Build history of the part. All positions in model axes, mm. A direction names the side the tool comes from. Coordinates: 2 decimals unless noted, no trailing zeros. Order: outer loops, then holes, each group sorted by start corner. A loop starts at its lowest first (then second) coordinate and runs counter-clockwise, first axis right, second up. Notation, with made-up numbers: (22, -4) - (63, -4) arc R23 cw to (63, 24) - close; hole circle Ø11 at (28.5, 77). An arc over 180 degrees is marked (long way). One line per item, written item: value.
from build123d import *

# Parameters (mm, degrees)
F0_R     = 5
F0_W     = 15
F0_H     = 22
F1_DEPTH = 2.5


with BuildPart() as f1:
    # F0 (on Top) → F1 (new body)
    with BuildSketch(Plane.XY):
        with BuildLine():
            Line((30, 57), (-30, 57))
            ThreePointArc((-30, 57), (-33.535534, 55.535534), (-35, 52))
            Line((-35, 52), (-35, -52))
            ThreePointArc((-35, -52), (-33.535534, -55.535534), (-30, -57))
            Line((-30, -57), (30, -57))
            ThreePointArc((30, -57), (33.535534, -55.535534), (35, -52))
            Line((35, -52), (35, 52))
            ThreePointArc((35, 52), (33.535534, 55.535534), (30, 57))
        make_face()
        with Locations((0, -50.2)):
            Circle(F0_R, mode=Mode.SUBTRACT)
        Rectangle(F0_W, F0_H, mode=Mode.SUBTRACT)
        with Locations((0, 50.2)):
            Circle(F0_R, mode=Mode.SUBTRACT)
    extrude(amount=F1_DEPTH)


solid = f1.part
1. Band-saw the part on A-A, the plane y = 50.2. Give the cut face in (x, z), and give its area (3 significant figures).
Values found:
outline: (-35, 0) - (-5, 0) - (-5, 2.5) - (-35, 2.5) - close; (5, 0) - (35, 0) - (35, 2.5) - (5, 2.5) - close
area: 150 mm2
2. Band-saw the part on B-B, the plane x = -3. Give the cut face in (y, z), and give its area (3 significant figures).
Values found:
outline: (-57, 0) - (-54.2, 0) - (-54.2, 2.5) - (-57, 2.5) - close; (-46.2, 0) - (-11, 0) - (-11, 2.5) - (-46.2, 2.5) - close; (11, 0) - (46.2, 0) - (46.2, 2.5) - (11, 2.5) - close; (54.2, 0) - (57, 0) - (57, 2.5) - (54.2, 2.5) - close
area: 190 mm2
3. 3-axis set-ups, long thin cutter, end or side, ignore diameter. For faces 4 (the face through (34, 55, 1)), 5 (the face through (0, 11, 1)): which of +Z, -Z, +X, -X, +Y, -Y reach the whole face in a straight line?
Values found:
face 4: +Z, -Z, +X, +Y
face 5: +Z, -Z
4. Band-saw the part on D-D, the plane y = -8.5. Give the cut face in (x, z).
Values found:
outline: (-35, 0) - (-7.5, 0) - (-7.5, 2.5) - (-35, 2.5) - close; (7.5, 0) - (35, 0) - (35, 2.5) - (7.5, 2.5) - close
5. Band-saw the part on C-C, the plane z = 1.1. Give the cut face in (x, y), and give its area (3 significant figures).
Values found:
outline: (-35, -52) arc R5 ccw to (-30, -57) - (30, -57) arc R5 ccw to (35, -52) - (35, 52) arc R5 ccw to (30, 57) - (-30, 57) arc R5 ccw to (-35, 52) - close; hole (-7.5, -11) - (7.5, -11) - (7.5, 11) - (-7.5, 11) - close; hole circle Ø10 at (0, -50.2); hole circle Ø10 at (0, 50.2)
area: 7,470 mm2
6. Probe line 1 along Y through (x, z) = (0, 0.7); line 2 along X through (y, z) = (-10.5, 1.7); line 3 along Y through (x, z) = (-4.5, 0.9). List the from-to ranges inside material, lowest first.
Values found:
line 1: y = -57 to -55.2, -45.2 to -11, 11 to 45.2, 55.2 to 57
line 2: x = -35 to -7.5, 7.5 to 35
line 3: y = -57 to -52.38, -48.02 to -11, 11 to 48.02, 52.38 to 57
7. Two-plate mould, pull along Y, no slides. Class faces 1 (the face through (7.5, 0, 1)), 2 (the face through (35, -1, 1)), 3 (the face through (0, -57, 1)): pulls with the +Y half, pulls with the -Y half, needs draft (parallel to the pull), parting line crosses it, or undercut.
Values found:
face 1: undercut
face 2: needs draft
face 3: pulls with the -Y half
